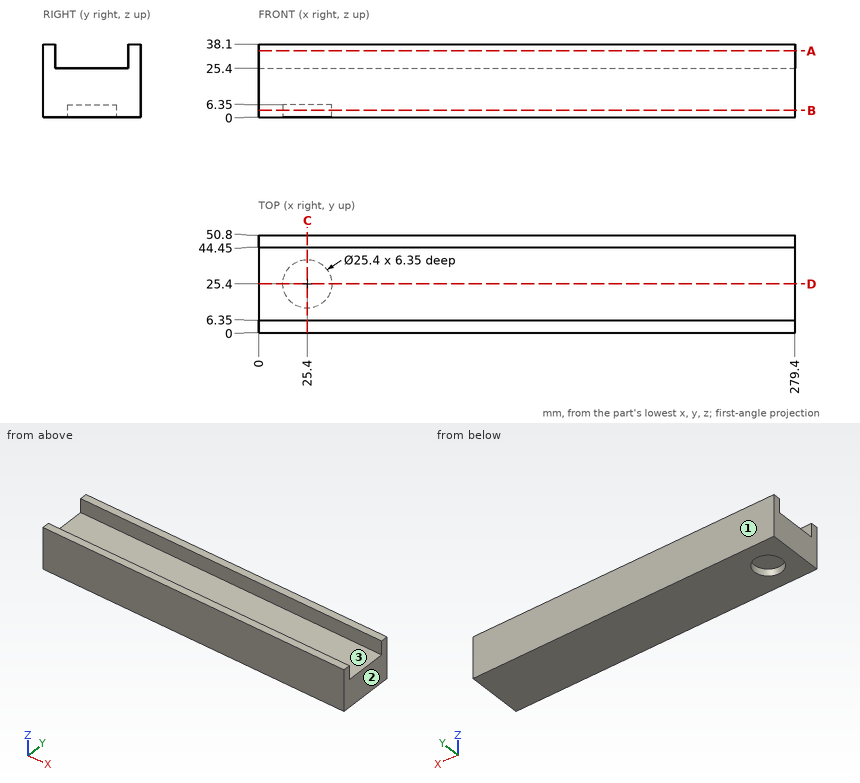
Drawing for the job (mm, zero at the part's lowest x, y, z). Give positions to 0.01 mm unless a question says otherwise; leave off trailing zeros. Loops run counter-clockwise (first coordinate to the right, second up) from the corner with the lowest first, then second, coordinate; pieces in that order, holes last. Notation, with made-up numbers: M 45,36.5 L 82,36.5 A18 ccw 82,47.5 Z; hole C 36,47 d1. An arc over 180 degrees is marked long. One line per question, with ' | ' between items. Start each with the question number.
1. Saw through at C-C on x = 25.4. Give the cut face in (y, z).
2. Saw through at D-D on y = 25.4. Give the cut face in (x, z).
3. Flat gauge pins, fed straight in: pin 1 (12 mm diameter, centred on x = 215, z = 27.5, fed in from -Y); pin 2 (5 mm diameter, centred on x = 54.5, y = 10.5, fed in from +Z). Where does each tip first touch, or does it go through?
4. Saw through at B-B on z = 3.5. Give the cut face in (x, y).
5. Probe L1, parallel to Y at x = 17, z = 35.5; L2, parallel to X at y = 25.4, z = 4.75; L3, parallel to Y at x = 25, z = 4. List the from-to ranges inside material, lowest first. Write a range as from..to.
6. Two-plate mould, pull along Y, no slides. Class the marked faces 1, 2 and 3: pulls with the +Y half, pulls with the -Y half, needs draft (parallel to the pull), parting line crosses it, or undercut.
7. Saw through at A-A on z = 34.5. Give the cut face in (x, y), plus the area to 3 significant figures.
Result sheet:
1) outline: M 0,0 L 12.7,0 L 12.7,6.35 L 38.1,6.35 L 38.1,0 L 50.8,0 L 50.8,38.1 L 44.45,38.1 L 44.45,25.4 L 6.35,25.4 L 6.35,38.1 L 0,38.1 Z
2) outline: M 0,0 L 12.7,0 L 12.7,6.35 L 38.1,6.35 L 38.1,0 L 279.4,0 L 279.4,25.4 L 0,25.4 Z
3) pin 1: stops at y = 0 | pin 2: stops at z = 25.4
4) outline: M 0,0 L 279.4,0 L 279.4,50.8 L 0,50.8 Z; hole C 25.4,25.4 d25.4
5) L1: y = 0..6.35, 44.45..50.8 | L2: x = 0..12.7, 38.1..279.4 | L3: y = 0..12.71, 38.09..50.8
6) face 1: pulls with the +Y half | face 2: needs draft | face 3: undercut
7) outline: M 0,0 L 279.4,0 L 279.4,6.35 L 0,6.35 Z; M 0,44.45 L 279.4,44.45 L 279.4,50.8 L 0,50.8 Z | area: 3,550 mm^2
